```python
from build123d import *

# Parameters (mm, degrees)
BOSS_EXTRUDE1_DEPTH = 20
SKETCH2_R           = 2
CUT_EXTRUDE1_DEPTH  = 40
SKETCH4_R           = 5.5
CUT_EXTRUDE2_DEPTH  = 1.75


with BuildPart() as part:
    # Sketch1 → Boss-Extrude1 (new body, symmetric)
    with BuildSketch(Plane.XY):
        Polygon((13, -4), (21, -4), (21, 4), (-21, 4), (-21, -4), (-13, -4), (-13, -16), (13, -16), align=None)
    extrude(amount=BOSS_EXTRUDE1_DEPTH, both=True)

    # Sketch2 → Cut-Extrude1 (cut)
    with BuildSketch(Plane(origin=(0, 4, 0), x_dir=(1, 0, 0), z_dir=(0, 1, 0))):
        with Locations((-16, 10)):
            Circle(SKETCH2_R)
        with Locations((16, 10)):
            Circle(SKETCH2_R)
        with Locations((-16, -10)):
            Circle(SKETCH2_R)
        with Locations((16, -10)):
            Circle(SKETCH2_R)
    extrude(amount=-CUT_EXTRUDE1_DEPTH, mode=Mode.SUBTRACT)

    # Sketch4 → Cut-Extrude2 (cut)
    with BuildSketch(Plane.XZ.offset(16)):
        with Locations((0, -4.5)):
            Circle(SKETCH4_R)
    extrude(amount=-CUT_EXTRUDE2_DEPTH, mode=Mode.SUBTRACT)


solid = part.part
```
Check sheet for the modelled part. Datum: model origin and axes. Units: mm. A direction names the side the tool comes from. Give positions to 0.01 mm unless a question says otherwise; leave off trailing zeros. Order: outer loops, then holes, each group sorted by start corner. A loop starts at its lowest first (then second) coordinate and runs counter-clockwise, first axis right, second up. Notation, with made-up numbers: M -3.75,83.25 L 26.25,83.25 A24 ccw 26.25,120.25 Z; hole C 86.5,89 d4. An arc over 180 degrees is marked long. Answer in a Markdown table with one row per item.
1) Release check for a two-part mould opening along Z. For faces 5 (the cylindrical face through (14.526, 0.056, 8.648)), 6 (the flat face through (-17, -4, 0)), 7 (the flat face through (0, -4, 20)), 8 (the cylindrical face through (-17.474, 0.056, -11.352)) record: +Z half, -Z half, draft (parallel to the pull), parting line (faces both ways), or undercut.
Filled sheet:
| item | result |
|---|---|
| face 5 | undercut |
| face 6 | draft |
| face 7 | +Z half |
| face 8 | undercut |
2) Cross-section at A-A, the plane x = -16. Enter the section's corners in (y, z), plus the area to 3 significant figures.
Filled sheet:
| item | result |
|---|---|
| outline | M -4,-20 L 4,-20 L 4,-12 L -4,-12 Z; M -4,-8 L 4,-8 L 4,8 L -4,8 Z; M -4,12 L 4,12 L 4,20 L -4,20 Z |
| area | 256 mm2 |
3) Thickness scan on L1, parallel to X at y = 0.5, z = 10; L2, parallel to X at y = -9, z = 3; L3, parallel to X at y = -1, z = -8.5. Record the ranges inside material, lowest first. Write a range as [from, to].
Filled sheet:
| item | result |
|---|---|
| L1 | x = [-21, -18], [-14, 14], [18, 21] |
| L2 | x = [-13, 13] |
| L3 | x = [-21, -17.32], [-14.68, 14.68], [17.32, 21] |
4) Access from +Z, -Z, +X, -X, +Y, -Y to the whole of each face (thin tool, end or side, straight path). Record for faces 1 (the flat face through (17, -4, 0)), 2 (the flat face through (-13, -10, 0)), 3 (the cylindrical face through (-1.19, -15.14, -9.87)), 4 (the flat face through (-21, 0, 0)).
Filled sheet:
| item | result |
|---|---|
| face 1 | +Z, -Z, +X, -Y |
| face 2 | +Z, -Z, -X, -Y |
| face 3 | -Y |
| face 4 | +Z, -Z, -X, +Y, -Y |
5) Cross-section at B-B, the plane z = 10. Enter the section's corners in (x, y), plus the area to 3 significant figures.
Filled sheet:
| item | result |
|---|---|
| outline | M -21,-4 L -18,-4 L -18,4 L -21,4 Z; M -14,-4 L -13,-4 L -13,-16 L 13,-16 L 13,-4 L 14,-4 L 14,4 L -14,4 Z; M 18,-4 L 21,-4 L 21,4 L 18,4 Z |
| area | 584 mm2 |
6) Gauge pin test, flat ends, axial feed: P1, Ø9, axis at x = 16.5, z = 4.5, coming from the -Y side; P2, Ø6.5, axis at x = -16.5, z = 10, coming from the -Y side; P3, Ø5, axis at y = -7.5, z = -1.5, coming from the -X side. Record the tip position at first contact, or that the pin passes through.
Filled sheet:
| item | result |
|---|---|
| P1 | stops at y = -16 |
| P2 | stops at y = -4 |
| P3 | stops at x = -13 |
7) Cross-section at D-D, the plane z = -14. Enter the section's corners in (x, y), plus the area to 3 significant figures.
Filled sheet:
| item | result |
|---|---|
| outline | M -21,-4 L -13,-4 L -13,-16 L 13,-16 L 13,-4 L 21,-4 L 21,4 L -21,4 Z |
| area | 648 mm2 |
8) Cross-section at C-C, the plane y = 0.5. Enter the section's corners in (x, z).
Filled sheet:
| item | result |
|---|---|
| outline | M -21,-20 L 21,-20 L 21,20 L -21,20 Z; hole C -16,-10 d4; hole C -16,10 d4; hole C 16,-10 d4; hole C 16,10 d4 |
